Verification items for this drawing (mm, ordinates from the low corner). A direction names the side the tool comes from. Coordinates: 2 decimals unless noted, no trailing zeros. Write each loop counter-clockwise with the first axis right and the second up, starting at its lowest first coordinate (ties: lowest second). Pieces come first, ordered by that corner, then holes. Notation, with made-up numbers: M 60,19 L 73,19 A20 ccw 73,54 Z; hole C 81,45.5 d2. An arc over 180 degrees is marked long. Write each question's results on one line, items separated by ' | '.
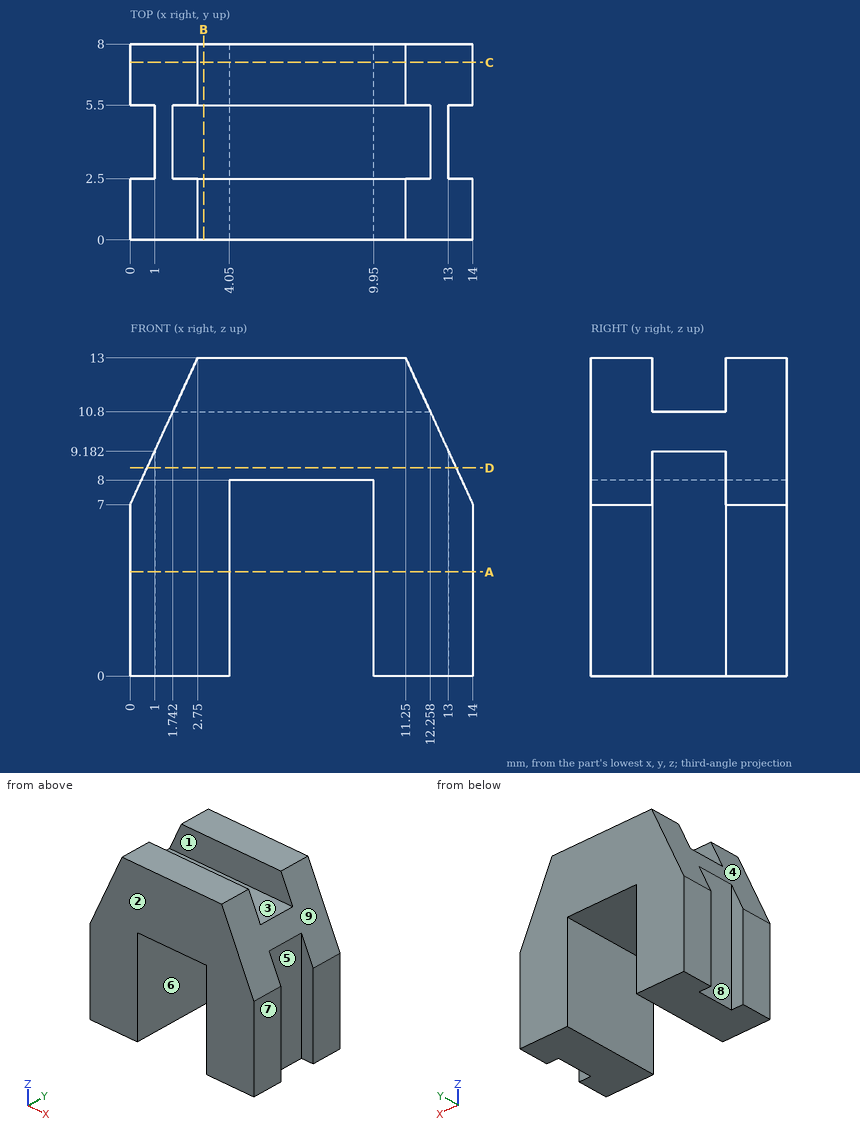
Q1. Mould release check, pull along Y, two halves, no side actions. Record for the marked faces 1, 2, 3 and 4: pulls with the +Y half, pulls with the -Y half, needs draft (parallel to the pull), parting line crosses it, or undercut.
Geometry check:
face 1: undercut | face 2: pulls with the -Y half | face 3: undercut | face 4: needs draft
Q2. Sectioned sample at A-A on z = 4.25. Record the cut outline in (x, y), and give its area (3 significant figures).
Geometry check:
outline: M 0,0 L 4.05,0 L 4.05,8 L 0,8 L 0,5.5 L 1,5.5 L 1,2.5 L 0,2.5 Z; M 9.95,0 L 14,0 L 14,2.5 L 13,2.5 L 13,5.5 L 14,5.5 L 14,8 L 9.95,8 Z | area: 58.8 mm2
Q3. Sectioned sample at D-D on z = 8.5. Record the cut outline in (x, y).
Geometry check:
outline: M 0.69,0 L 13.31,0 L 13.31,2.5 L 13,2.5 L 13,5.5 L 13.31,5.5 L 13.31,8 L 0.69,8 L 0.69,5.5 L 1,5.5 L 1,2.5 L 0.69,2.5 Z
Q4. Sectioned sample at B-B on x = 3. Record the cut outline in (y, z).
Geometry check:
outline: M 0,0 L 8,0 L 8,13 L 5.5,13 L 5.5,10.8 L 2.5,10.8 L 2.5,13 L 0,13 Z
Q5. Sectioned sample at C-C on y = 7.25. Record the cut outline in (x, z).
Geometry check:
outline: M 0,0 L 4.05,0 L 4.05,8 L 9.95,8 L 9.95,0 L 14,0 L 14,7 L 11.25,13 L 2.75,13 L 0,7 Z
Q6. Depth check by flat-ended pin: P1, Ø2.5, axis at x = 5.5, y = 4, coming from the +Z side; P2, Ø1.8, axis at x = 7.5, y = 4, coming from the -Z side; P3, Ø2.5, axis at y = 4, z = 6, coming from the +X side. Enter the tip coordinate at first touch or a pass-through.
Geometry check:
P1: stops at z = 10.8 | P2: stops at z = 8 | P3: stops at x = 13
Q7. Access from +Z, -Z, +X, -X, +Y, -Y to the whole of each face (thin tool, end or side, straight path). Record for the marked faces 5, 6, 7, 8 and 9.
Geometry check:
face 5: +Z, -Z, +X | face 6: -Z, +Y, -Y | face 7: +Z, -Z, +X, +Y, -Y | face 8: +Z, -Z, -X | face 9: +Z, +X, +Y, -Y
Q8. Scan lines: probe 1 along X at (y, z) = (7.25, 5.5); probe 2 along X at (y, z) = (3.75, 3.25); probe 3 along Y at (x, z) = (11.5, 11.5). Record each from-to range of solid material in increasing order.
Geometry check:
probe 1: x = 0 to 4.05, 9.95 to 14 | probe 2: x = 1 to 4.05, 9.95 to 13 | probe 3: y = 0 to 2.5, 5.5 to 8
